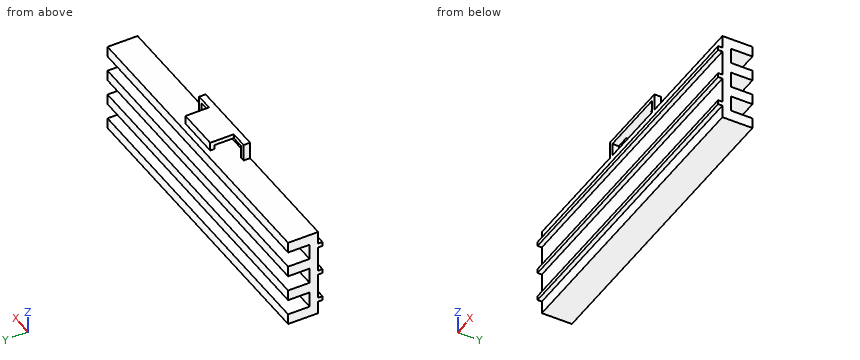
from build123d import *

# Parameters (mm, degrees)
BOSS_EXTRUDE1_DEPTH = 36.5
EXTRUDE_THIN1_DEPTH = 1.5
EXTRUDE_THIN2_DEPTH = 5


with BuildPart() as part:
    # Sketch1 → Boss-Extrude1 (new, symmetric)
    with BuildSketch(Plane(origin=(0, 0, 0), x_dir=(0, 0, -1), z_dir=(1, 0, 0))):
        Polygon((0.5, 0), (-0.5, 0), (-0.5, 1), (-6.5, 1), (-6.5, 0), (-7.5, 0), (-7.5, 1), (-10.5, 1), (-10.5, 8), (-8, 8), (-8, 3), (-4.333333333, 3), (-4.333333333, 8), (-1.833333333, 8), (-1.833333333, 3), (1.833333333, 3), (1.833333333, 8), (4.333333333, 8), (4.333333333, 3), (8, 3), (8, 8), (10.5, 8), (10.5, 1), (7.5, 1), (7.5, 0), (6.5, 0), (6.5, 1), (0.5, 1), align=None)
    extrude(amount=BOSS_EXTRUDE1_DEPTH, both=True)

    # Sketch3 → Extrude-Thin1 (add)
    with BuildSketch(Plane(origin=(0, 1, 0), x_dir=(1, 0, 0), z_dir=(0, 1, 0))):
        Polygon((-9, -10.5), (-9, -14.5), (9, -14.5), (9, -10.5), (8, -10.5), (8, -13.5), (-8, -13.5), (-8, -10.5), align=None)
    extrude(amount=EXTRUDE_THIN1_DEPTH)

    # Sketch4 → Extrude-Thin2 (add, symmetric)
    with BuildSketch(Plane(origin=(0, 0, 0), x_dir=(0, 0, -1), z_dir=(1, 0, 0))):
        Polygon((-14.5, 2.5), (-14.5, 8), (-12.5, 8), (-12.5, 7), (-13.5, 7), (-13.5, 2.5), align=None)
    extrude(amount=EXTRUDE_THIN2_DEPTH, both=True)


solid = part.part
Here's how the part is built. I have some questions about the finished solid (model axes, mm). Round coordinates to 2 decimals unless told otherwise and drop trailing zeros. Write each loop counter-clockwise with the first axis right and the second up, starting at its lowest first coordinate (ties: lowest second). Pieces come first, ordered by that corner, then holes.
1. Suppose I cut it at C-C (y = 3.75). List the corners of the cut face in (x, z) for me, and give its area (3 significant figures).
2. Suppose I cut it at A-A (z = 11.75). List the corners of the cut face in (x, y) for me, and give its area (3 significant figures).
3. Suppose I cut it at D-D (x = -12.5). List the corners of the cut face in (y, z) for me.
4. Will these pins go through, and if not, where does the flat tip stop? pin 1 Ø0.8 at (x, y) = (0.5, 0.5) entering from -Z; pin 2 Ø1.6 at (y, z) = (1.5, 12.5) entering from -X; pin 3 Ø0.8 at (x, z) = (1, 13) entering from -Y.
5. I need wall thicknesses on L1, parallel to Z at x = 17.5, y = 6.25; L2, parallel to Z at x = -1, y = 4.5; L3, parallel to X at y = 7.75, z = 13.5. Which ranges of each line are inside material? Lowest first, please.
Answer sheet:
1. outline: (-36.5, -10.5) - (36.5, -10.5) - (36.5, -8) - (-36.5, -8) - close; (-36.5, -4.33) - (36.5, -4.33) - (36.5, -1.83) - (-36.5, -1.83) - close; (-36.5, 1.83) - (36.5, 1.83) - (36.5, 4.33) - (-36.5, 4.33) - close; (-36.5, 8) - (36.5, 8) - (36.5, 10.5) - (-36.5, 10.5) - close; (-5, 13.5) - (5, 13.5) - (5, 14.5) - (-5, 14.5) - close
1. area: 740 mm2
2. outline: (-9, 1) - (-8, 1) - (-8, 2.5) - (-9, 2.5) - close; (8, 1) - (9, 1) - (9, 2.5) - (8, 2.5) - close
2. area: 3.00 mm2
3. outline: (0, -7.5) - (1, -7.5) - (1, -10.5) - (8, -10.5) - (8, -8) - (3, -8) - (3, -4.33) - (8, -4.33) - (8, -1.83) - (3, -1.83) - (3, 1.83) - (8, 1.83) - (8, 4.33) - (3, 4.33) - (3, 8) - (8, 8) - (8, 10.5) - (1, 10.5) - (1, 7.5) - (0, 7.5) - (0, 6.5) - (1, 6.5) - (1, 0.5) - (0, 0.5) - (0, -0.5) - (1, -0.5) - (1, -6.5) - (0, -6.5) - close
4. pin 1: stops at z = -7.5
4. pin 2: stops at x = -9
4. pin 3: stops at y = 7
5. L1: z = -10.5 to -8, -4.33 to -1.83, 1.83 to 4.33, 8 to 10.5
5. L2: z = -10.5 to -8, -4.33 to -1.83, 1.83 to 4.33, 8 to 10.5, 13.5 to 14.5
5. L3: x = -5 to 5
